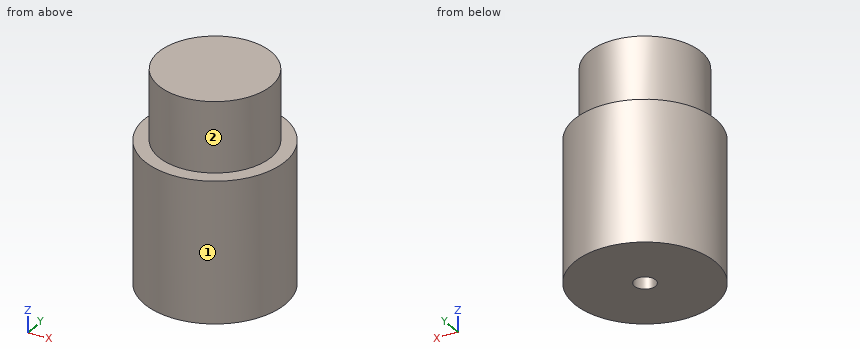
from build123d import *

# Parameters (mm, degrees)
SKETCH_1_R          = 10
EXTRUDE_1_DEPTH     = 20
SKETCH_2_R          = 1.5
CUT_EXTRUDE_1_DEPTH = 10
SKETCH_3_R          = 8
EXTRUDE_2_DEPTH     = 10


with BuildPart() as part:
    # 스케치1 → 보스-돌출1 (new body)
    with BuildSketch(Plane.XY):
        Circle(SKETCH_1_R)
    extrude(amount=EXTRUDE_1_DEPTH)

    # 스케치2 → 컷-돌출1 (cut)
    with BuildSketch(Plane(origin=(0, 0, 0), x_dir=(-1, 0, 0), z_dir=(0, 0, -1))):
        Circle(SKETCH_2_R)
    extrude(amount=-CUT_EXTRUDE_1_DEPTH, mode=Mode.SUBTRACT)

    # 스케치3 → 보스-돌출2 (add)
    with BuildSketch(Plane.XY.offset(20)):
        Circle(SKETCH_3_R)
    extrude(amount=EXTRUDE_2_DEPTH)


solid = part.part
Work out the finished part from the listing and answer in its coordinate system (mm). Face numbers are marked on the shaded views. A direction names the side the tool comes from. Coordinates: 2 decimals unless noted, no trailing zeros. Loops run counter-clockwise (first coordinate to the right, second up) from the corner with the lowest first, then second, coordinate; pieces in that order, holes last. Notation, with made-up numbers: M 76.25,62.25 L 94.25,62.25 A19 cw 94.25,86.25 Z; hole C 59.25,22.5 d3. An arc over 180 degrees is marked long. Answer in a Markdown table with one row per item. Add a question column.
1. Flat-ended cylindrical pins translate along their axes: P1, Ø2, axis at y = 6.5, z = 24.5, coming from the +X side; P2, Ø4, axis at x = 7.5, z = 7, coming from the +Y side; P3, Ø0.9, axis at x = 0, y = -0.5, coming from the -Z side. Find the tip coordinate at first contact, or state that the pin passes through.
2. Find section C-C, the plane z = 9.5. Write down the section's boundary in (x, y).
3. Find section D-D, the plane x = -2.5. Write down the section's boundary in (y, z), then the cut area to 3 significant figures.
4. Consider L1, parallel to Y at x = 0, z = 6; L2, parallel to Z at x = 8.25, y = -5.25; L3, parallel to Y at x = -0.25, z = 18.5. Determine where each line is inside the solid, lowest interval first.
5. A tool of negligible diameter and unlimited length cuts with its end or side. For the marked faces 1 and 2, from which of +Z, -Z, +X, -X, +Y, -Y can it reach the whole face along a straight path? Write none if from no direction.
6. Find section A-A, the plane y = 0. Write down the section's boundary in (x, z), then the cut area to 3 significant figures.
Reported:
| question | item | result |
|---|---|---|
| 1 | P1 | stops at x = 5.81 |
| 1 | P2 | stops at y = 8.35 |
| 1 | P3 | stops at z = 10 |
| 2 | outline | C 0,0 d20; hole C 0,0 d3 |
| 3 | outline | M -9.68,0 L 9.68,0 L 9.68,20 L 7.6,20 L 7.6,30 L -7.6,30 L -7.6,20 L -9.68,20 Z |
| 3 | area | 539 mm^2 |
| 4 | L1 | y = -10 to -1.5, 1.5 to 10 |
| 4 | L2 | z = 0 to 20 |
| 4 | L3 | y = -10 to 10 |
| 5 | face 1 | +Z, -Z |
| 5 | face 2 | +Z |
| 6 | outline | M -10,0 L -1.5,0 L -1.5,10 L 1.5,10 L 1.5,0 L 10,0 L 10,20 L 8,20 L 8,30 L -8,30 L -8,20 L -10,20 Z |
| 6 | area | 530 mm^2 |
